Autodesk Inventor part; units mm, degrees
ref_plane "YZ Plane" through (0, 0, 0) normal (1, 0, 0) x (0, 1, 0)
ref_plane "XZ Plane" through (0, 0, 0) normal (0, 1, 0) x (-1, 0, 0)
ref_plane "XY Plane" through (0, 0, 0) normal (0, 0, 1) x (1, 0, 0)
ref_plane "Work Plane1" through (0, 0, 0) normal (0, 0, 1) x (1, 0, 0)
sketch "Sketch1" plane through (0, 0, 0) normal (0, 0, 1) x (1, 0, 0)
  line L0 (-17.7099, -6.35) -> (57.15, -6.35)
  line L1 (57.15, 0) -> (-17.7099, 0)
  line L2 (1.3284, -28.575) -> (1.3284, 22.225)
  line L3 (1.3284, -28.575) -> (7.6784, -28.575)
  line L4 (7.6784, 22.225) -> (7.6784, -28.575)
  line L5 (1.3284, 22.225) -> (7.6784, 22.225)
  line L6 (63.5, -28.575) -> (63.5, 22.225)
  line L7 (63.5, 22.225) -> (57.15, 22.225)
  line L8 (57.15, -28.575) -> (57.15, 22.225)
  line L9 (63.5, -28.575) -> (57.15, -28.575)
  line L10 (7.6835, 0) -> (57.15, 0)
  line L11 (57.15, 0) -> (57.15, 25.4)
  line L12 (57.15, 25.4) -> (7.6835, 25.4)
  line L13 (7.6835, 25.4) -> (7.6835, 0)
  circle A0 centre (14.5257, 3.9217) radius 2.3813
  line L14 (32.4168, 24.8107) -> (32.4168, 0) construction
  circle A1 centre (50.3079, 3.9217) radius 2.3813
  line L15 (7.6835, 11.1252) -> (57.15, 11.1252) construction
  circle A2 centre (14.5257, 18.3287) radius 2.3813
  circle A3 centre (50.3079, 18.3287) radius 2.3813
  line L16 (57.15, 0) -> (57.15, -6.35)
  line L17 (-17.7099, 0) -> (-17.7099, -6.35)
  line L18 (57.15, 0) -> (63.5, 0)
  point P0 (0, 0)
  dimension "d0" = 4.7625
  dimension "d3" = 25.4
  dimension "d4" = 11.1252
extrude "Extrusion1" add sketch "Sketch1" against normal blind 6.35 contours L1 L13 L12 L11 L8 | A0 | A1
properties part number "basePlate01"
Input: part model. Units: mm. Frame: model coordinates. Coordinates: 2 decimals unless noted, no trailing zeros. Loops run counter-clockwise (first coordinate to the right, second up) from the corner with the lowest first, then second, coordinate; pieces in that order, holes last.
(1) Section A-A on y = 17.25. Return the cut outline in (x, z).
(2) Section B-B on x = 14. Return the cut outline in (y, z).
(3) Section C-C on z = -1.5. Return the cut outline in (x, y).
(4) Material intervals for probe 1 along X at (y, z) = (19.25, -5.25); probe 2 along X at (y, z) = (19.75, -4); probe 3 along Y at (x, z) = (49, -1.5), sorted ascending.
(5) Pull-direction query (Y, two-part tool) for faces 1 (the face through (33, 25.4, -3)), 2 (the face through (32, 13, 0)), 3 (the face through (16.8, 19.04, -3.13)); classes: released by +Y, released by -Y, zero draft, split by the parting line, or undercut.
Data:
1. outline: (7.68, -6.35) - (12.4, -6.35) - (12.4, 0) - (7.68, 0) - close; (16.65, -6.35) - (48.18, -6.35) - (48.18, 0) - (16.65, 0) - close; (52.43, -6.35) - (57.15, -6.35) - (57.15, 0) - (52.43, 0) - close
2. outline: (0, -6.35) - (16.01, -6.35) - (16.01, 0) - (0, 0) - close; (20.65, -6.35) - (25.4, -6.35) - (25.4, 0) - (20.65, 0) - close
3. outline: (7.68, 0) - (57.15, 0) - (57.15, 25.4) - (7.68, 25.4) - close; hole circle Ø4.76 at (14.53, 18.33); hole circle Ø4.76 at (50.31, 18.33)
4. probe 1: x = 7.68 to 12.33, 16.72 to 48.11, 52.5 to 57.15
4. probe 2: x = 7.68 to 12.62, 16.44 to 48.4, 52.22 to 57.15
4. probe 3: y = 0 to 16.34, 20.32 to 25.4
5. face 1: released by +Y
5. face 2: zero draft
5. face 3: undercut
